Solid Edge part; units mm, degrees
sketch "Sketch1" plane through (0, 0, 0) normal (0, 0, 1) x (1, 0, 0)
  line L0 (-19, -15) -> (19, -15)
  line L1 (19, -15) -> (19, 15)
  line L2 (19, 15) -> (-19, 15)
  line L3 (-19, 15) -> (-19, -15)
  dimension "D1" = 19
  dimension "D2" = 19
extrude "Protrusion1" add sketch "Sketch1" along normal blind 5
sketch "Sketch2" plane through (-19, 0, 2.5) normal (-1, 0, 0) x (0, -1, 0)
  circle A0 centre (-8.5, 0) radius 1.25
  circle A1 centre (8.5, 0) radius 1.25
extrude "ExtrudedCutout_1" cut sketch "Sketch2" against normal blind 6
mirror "Mirror1" about plane through (0, 0, 0) normal (1, 0, 0) of "ExtrudedCutout_1"
sketch "Sketch3" plane through (0, 0, 5) normal (0, 0, 1) x (1, 0, 0)
  circle A0 centre (0, 0) radius 2
extrude "ExtrudedCutout_2" cut sketch "Sketch3" against normal blind 3
sketch "Sketch4" plane through (0, 0, 0) normal (0, 0, -1) x (1, 0, 0)
  circle A0 centre (0, 0) radius 1.25
extrude "Cutout1" cut sketch "Sketch4" against normal through all
properties material "ABS Plastic, medium impact"
Check sheet for the modelled part. Datum: model origin and axes. Units: mm. A direction names the side the tool comes from. Round coordinates to 2 decimals unless told otherwise and drop trailing zeros. Write each loop counter-clockwise with the first axis right and the second up, starting at its lowest first coordinate (ties: lowest second). Pieces come first, ordered by that corner, then holes. Notation, with made-up numbers: (67, 29) - (110, 29) arc R36 cw to (110, 63) - close; hole circle Ø1 at (34.5, 57.25). An arc over 180 degrees is marked (long way). Return JSON: item names as keys, results as strings.
Q1. Depth check by flat-ended pin: P1, Ø3, axis at y = -8.5, z = 2.5, coming from the -X side; P2, Ø0.8, axis at y = -8.5, z = 2.5, coming from the -X side; P3, Ø3, axis at x = 0, y = 0, coming from the +Z side; P4, Ø0.8, axis at y = 8.5, z = 2, coming from the +X side. Enter the tip coordinate at first touch or a pass-through.
Returned:
{"P1": "stops at x = -19", "P2": "stops at x = -13", "P3": "stops at z = 2", "P4": "stops at x = 13"}
Q2. Cross-section at B-B (z = 3.25). Record the boundary of the cut face in (x, y), then the cut area to 3 significant figures.
Returned:
{"outline": "(-19, -15) - (19, -15) - (19, -9.5) - (13, -9.5) - (13, -7.5) - (19, -7.5) - (19, 7.5) - (13, 7.5) - (13, 9.5) - (19, 9.5) - (19, 15) - (-19, 15) - (-19, 9.5) - (-13, 9.5) - (-13, 7.5) - (-19, 7.5) - (-19, -7.5) - (-13, -7.5) - (-13, -9.5) - (-19, -9.5) - close; hole circle Ø4 at (0, 0)", "area": "1,080 mm²"}
Q3. Access from +Z, -Z, +X, -X, +Y, -Y to the whole of each face (thin tool, end or side, straight path). Record for faces 5 (the flat face through (0, 4, 0)), 6 (the flat face through (19, 0, 2)), 7 (the flat face through (13, -9, 2)), 8 (the cylindrical face through (-16.04, -7.25, 2.55)), 9 (the cylindrical face through (0, -2, 4)).
Returned:
{"face 5": "-Z, +X, -X, +Y, -Y", "face 6": "+Z, -Z, +X, +Y, -Y", "face 7": "+X", "face 8": "-X", "face 9": "+Z"}
Q4. Cross-section at A-A (y = 0). Record the boundary of the cut face in (x, z), then the cut area to 3 significant figures.
Returned:
{"outline": "(-19, 0) - (-1.25, 0) - (-1.25, 2) - (-2, 2) - (-2, 5) - (-19, 5) - close; (1.25, 0) - (19, 0) - (19, 5) - (2, 5) - (2, 2) - (1.25, 2) - close", "area": "173 mm²"}
Q5. Cross-section at D-D (y = -8.5). Record the boundary of the cut face in (x, z), then the cut area to 3 significant figures.
Returned:
{"outline": "(-19, 0) - (19, 0) - (19, 1.25) - (13, 1.25) - (13, 3.75) - (19, 3.75) - (19, 5) - (-19, 5) - (-19, 3.75) - (-13, 3.75) - (-13, 1.25) - (-19, 1.25) - close", "area": "160 mm²"}
Q6. Scan lines: L1, parallel to Y at x = 0, z = 0.75; L2, parallel to Z at x = -14.25, y = 8.5; L3, parallel to X at y = 0, z = 1.4. Record each from-to range of solid material in increasing order. Write a range as from..to.
Returned:
{"L1": "y = -15..-1.25, 1.25..15", "L2": "z = 0..1.25, 3.75..5", "L3": "x = -19..-1.25, 1.25..19"}
Q7. Draft check along Z on faces 1 (the flat face through (0, 15, 2)), 2 (the cylindrical face through (16.04, 9.75, 2.45)), 3 (the flat face through (0, 4, 5)), 4 (the cylindrical face through (16.04, -7.25, 2.45)). Enter one of: released by +Z, released by -Z, zero draft, split by the parting line, or undercut.
Returned:
{"face 1": "zero draft", "face 2": "undercut", "face 3": "released by +Z", "face 4": "undercut"}
Q8. Cross-section at C-C (x = -17). Record the boundary of the cut face in (y, z), then the cut area to 3 significant figures.
Returned:
{"outline": "(-15, 0) - (15, 0) - (15, 5) - (-15, 5) - close; hole circle Ø2.5 at (-8.5, 2.5); hole circle Ø2.5 at (8.5, 2.5)", "area": "140 mm²"}
